Input: dimensioned drawing with shaded views. Units: mm. Origin: part minimum x, y, z. A direction names the side the tool comes from. Give positions to 0.01 mm unless a question says otherwise; leave off trailing zeros. Write each loop counter-clockwise with the first axis right and the second up, starting at its lowest first coordinate (ties: lowest second). Pieces come first, ordered by that corner, then holes. Notation, with made-up numbers: (60.25, -26.75) -> (68.25, -26.75) arc R24 cw to (68.25, -16.75) -> close; hole circle Ø7 at (67.25, -14.5). An arc over 180 degrees is marked (long way). Answer as a JSON object with one key per item and string values. Group by question number.
(1) Section query A-A on y = 22.5. Output: boundary loops of the cut face in (x, z).
(2) Section query D-D on x = 11.25. Output: boundary loops of the cut face in (y, z) (1 decimal).
(3) Section query B-B on x = 7.94. State how many separate pieces and enclosed holes the cut face has.
(4) Set-up query: the marked faces 1, 2 and 3. Return all of +Z, -Z, +X, -X, +Y, -Y with unobstructed straight access to the full face (end or side cutting, diameter ignored); none if empty.
(5) Material intervals for probe 1 along Y at (x, z) = (7.94, 2.2); probe 2 along X at (y, z) = (41.55, 1.75); probe 3 along X at (y, z) = (28, 10), sorted ascending.
(6) Section query C-C on z = 22.5. Output: boundary loops of the cut face in (x, y).
(7) Contact query for flat-ended pins moving along their axis: pin 1 Ø3 at (x, z) = (6.5, 20.5) entering from -Y; pin 2 Ø1.5 at (x, y) = (2, 25.5) entering from +Z (1 decimal); pin 3 Ø6 at (y, z) = (7.5, 19.5) entering from -X. Output: stop coordinate, or through.
(8) Draft query along Y for the marked faces 4, 5 and 6. Return one class per face: +Y half, -Y half, draft (parallel to the pull), parting line (faces both ways), or undercut.
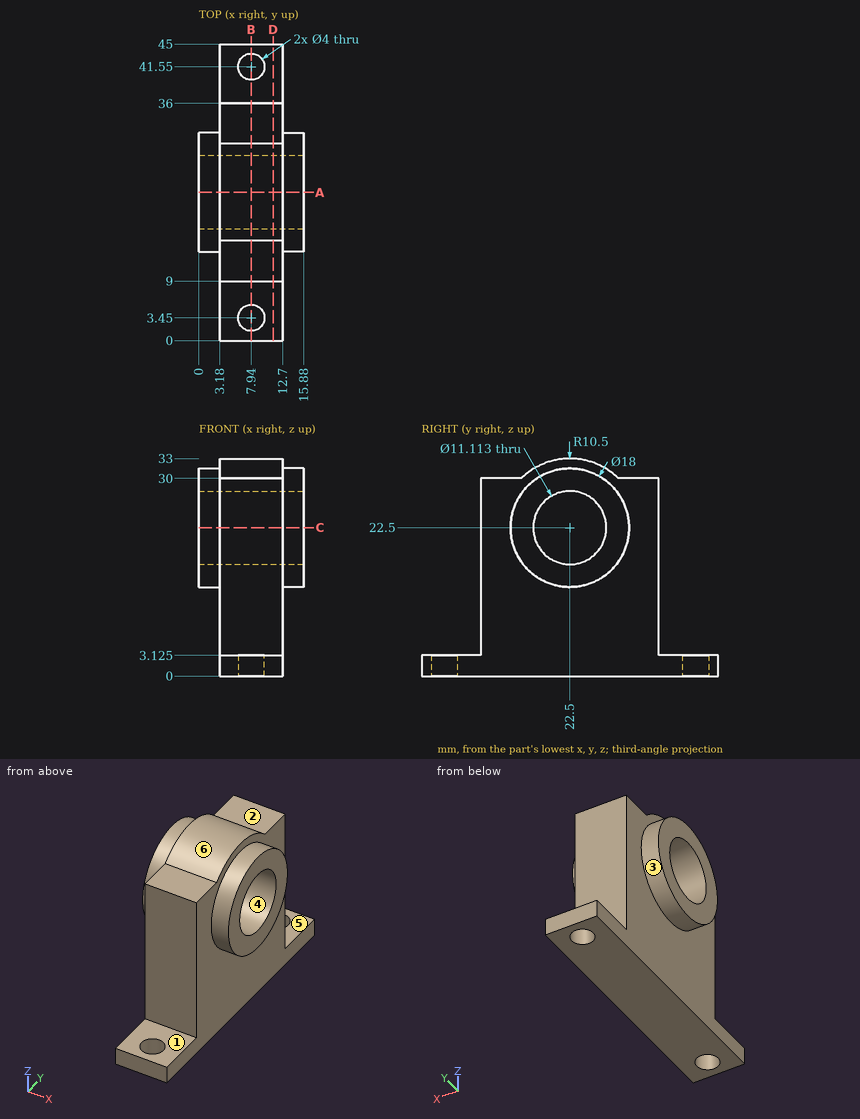
Answer list:
{
 "1": {"outline": "(0, 13.5) -> (3.18, 13.5) -> (3.18, 0) -> (12.7, 0) -> (12.7, 13.5) -> (15.88, 13.5) -> (15.88, 16.94) -> (0, 16.94) -> close; (0, 28.06) -> (15.88, 28.06) -> (15.88, 31.5) -> (12.7, 31.5) -> (12.7, 33) -> (3.18, 33) -> (3.18, 31.5) -> (0, 31.5) -> close"},
 "2": {"outline": "(0, 0) -> (45, 0) -> (45, 3.1) -> (36, 3.1) -> (36, 30) -> (29.8, 30) arc R10.5 ccw to (15.2, 30) -> (9, 30) -> (9, 3.1) -> (0, 3.1) -> close; hole circle Ø11.1 at (22.5, 22.5)"},
 "3": {"separate pieces": "3", "enclosed holes": "1"},
 "4": {"face 1": "+Z, +X, -X, -Y", "face 2": "+Z, +X, -X, +Y", "face 3": "-X"},
 "5": {"probe 1": "0 to 1.45, 5.45 to 39.55, 43.55 to 45", "probe 2": "3.18 to 5.94, 9.94 to 12.7", "probe 3": "3.18 to 12.7"},
 "6": {"outline": "(0, 13.5) -> (3.18, 13.5) -> (3.18, 9) -> (12.7, 9) -> (12.7, 13.5) -> (15.88, 13.5) -> (15.88, 16.94) -> (0, 16.94) -> close; (0, 28.06) -> (15.88, 28.06) -> (15.88, 31.5) -> (12.7, 31.5) -> (12.7, 36) -> (3.18, 36) -> (3.18, 31.5) -> (0, 31.5) -> close"},
 "7": {"pin 1": "y = 9", "pin 2": "z = 31.2", "pin 3": "x = 3.18"},
 "8": {"face 4": "undercut", "face 5": "draft", "face 6": "parting line"}
}
